```python
from build123d import *

# Parameters (mm, degrees)
F0_W      = 79.3684571981
F0_H      = 71.8531981111
F1_DEPTH  = 25.4
F2_DEPTH  = 25.4
F4_DEPTH  = 101.6
F5_R      = 4.7587178315
F6_DEPTH  = 127
F7_DEPTH  = 508
F9_DEPTH  = 7.62
F11_DEPTH = 25.4
F12_DEPTH = 12.7


with BuildPart() as f1:
    # F0 (on Top) → F1 (new body)
    with BuildSketch(Plane.XY):
        Rectangle(F0_W, F0_H)
    extrude(amount=F1_DEPTH)

    # F2 (add): a face of the model
    f2_faces = [f1.faces().sort_by_distance(p)[0] for p in [
        (0, 0, 25.4),
    ]]
    extrude(f2_faces, amount=F2_DEPTH)

    # F3 (on face) → F4 (cut)
    with BuildSketch(Plane.XZ.offset(35.9265990555)):
        with BuildLine():
            ThreePointArc((-17.4702548625, 50.8), (0, 33.3297451375), (17.4702548625, 50.8))
            Line((17.4702548625, 50.8), (-17.4702548625, 50.8))
        make_face()
    extrude(amount=-F4_DEPTH, mode=Mode.SUBTRACT)

    # F5 (on face) → F6 (join)
    with BuildSketch(Plane.XY.offset(50.8)):
        with Locations((-29.7860819846, 0)):
            Circle(F5_R)
        with Locations((28.1363911927, 0)):
            Circle(F5_R)
    extrude(amount=F6_DEPTH)

    # F7 (cut): faces of the model
    f7_faces = [f1.faces().sort_by_distance(p)[0] for p in [
        (28.1363911927, 0, 177.8),
        (-29.7860819846, 0, 177.8),
    ]]
    extrude(f7_faces, amount=-F7_DEPTH, mode=Mode.SUBTRACT)

    # F8 (on face) → F9 (join)
    with BuildSketch(Plane.XZ.offset(35.9265990555)):
        with BuildLine():
            Line((-17.4702548625, 50.8), (-22.6149617575, 50.8))
            ThreePointArc((-22.6149617575, 50.8), (0, 28.1850382425), (22.6149617575, 50.8))
            Line((22.6149617575, 50.8), (17.4702548625, 50.8))
            ThreePointArc((17.4702548625, 50.8), (0, 33.3297451375), (-17.4702548625, 50.8))
        make_face()
    extrude(amount=F9_DEPTH)

    # F10 (on face) → F11 (join)
    with BuildSketch(Plane(origin=(0, 35.9265990555, 0), x_dir=(-1, 0, 0), z_dir=(0, 1, 0))):
        with BuildLine():
            Line((-17.4702548625, 50.8), (-23.0630593563, 50.8))
            ThreePointArc((-23.0630593563, 50.8), (0, 27.7369406437), (23.0630593563, 50.8))
            Line((23.0630593563, 50.8), (17.4702548625, 50.8))
            ThreePointArc((17.4702548625, 50.8), (0, 33.3297451375), (-17.4702548625, 50.8))
        make_face()
    extrude(amount=F11_DEPTH)

    # F12 (cut): a face of the model
    f12_faces = [f1.faces().sort_by_distance(p)[0] for p in [
        (20.2666571094, 61.3265990555, 50.2842943151),
    ]]
    extrude(f12_faces, amount=-F12_DEPTH, mode=Mode.SUBTRACT)


solid = f1.part
```
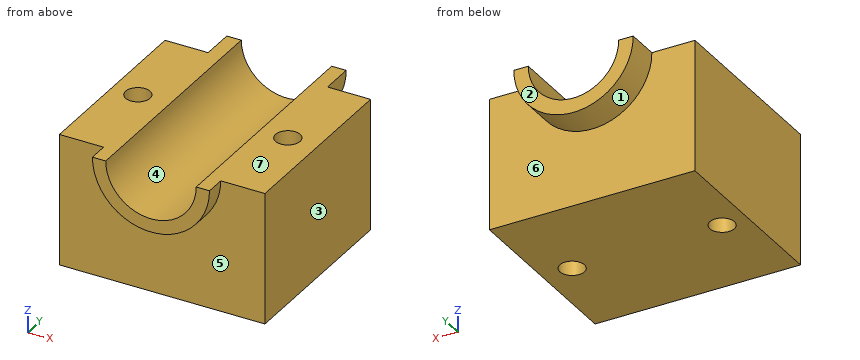
Check sheet for the modelled part. Datum: model origin and axes. Units: mm. Face numbers are marked on the shaded views. A direction names the side the tool comes from. Coordinates: 2 decimals unless noted, no trailing zeros. Order: outer loops, then holes, each group sorted by start corner. A loop starts at its lowest first (then second) coordinate and runs counter-clockwise, first axis right, second up. Notation, with made-up numbers: M 20,82 L 56,82 A10 ccw 56,97 Z; hole C -14,9.25 d5. An arc over 180 degrees is marked long. One line per question, with ' | ' between items. Start each with the question number.
Item 1: Access from +Z, -Z, +X, -X, +Y, -Y to the whole of each face (thin tool, end or side, straight path). Record for the marked faces 5, 6 and 7.
Item 2: Sectioned sample at A-A on y = 0. Record the cut outline in (x, z).
Item 3: Gauge pin test, flat ends, axial feed: P1, Ø15, axis at x = 14.5, z = 13, coming from the +Y side; P2, Ø1.5, axis at x = -30, z = 35, coming from the -Y side. Record the tip position at first contact, or that the pin passes through.
Item 4: Sectioned sample at D-D on x = -6. Record the cut outline in (y, z), and give its area (3 significant figures).
Item 5: Material ranges on line 1 (Y direction, x = -6, z = 19); line 2 (X direction, y = 45, z = 41.5); line 3 (X direction, y = -29.5, z = 38), recorded low to high.
Item 6: Sectioned sample at B-B on z = 38. Record the cut outline in (x, y), and give its area (3 significant figures).
Item 7: Sectioned sample at C-C on y = -34.5. Record the cut outline in (x, z), and give its area (3 significant figures).
Item 8: Mould release check, pull along X, two halves, no side actions. Record for the marked faces 1, 2, 3 and 4: pulls with the +X half, pulls with the -X half, needs draft (parallel to the pull), parting line crosses it, or undercut.
Answer below:
1) face 5: -Z, -Y | face 6: -Z, +Y | face 7: +Z, +X, -X, +Y, -Y
2) outline: M -39.68,0 L -34.54,0 L -34.54,50.8 L -39.68,50.8 Z; M -25.03,0 L 23.38,0 L 23.38,50.8 L 17.47,50.8 A17.47 cw -17.47,50.8 L -25.03,50.8 Z; M 32.9,0 L 39.68,0 L 39.68,50.8 L 32.9,50.8 Z
3) P1: stops at y = 35.93 | P2: stops at y = -35.93
4) outline: M -43.55,29 L -35.93,29 L -35.93,0 L 35.93,0 L 35.93,28.53 L 48.63,28.53 L 48.63,34.39 L -43.55,34.39 Z | area: 2,590 mm^2
5) line 1: y = -35.93 to 35.93 | line 2: x = -21.1 to -14.79, 14.79 to 21.1 | line 3: x = -39.68 to -11.89, 11.89 to 39.68
6) outline: M -39.68,-35.93 L -18.64,-35.93 L -18.64,-43.55 L -11.89,-43.55 L -11.89,48.63 L -19.19,48.63 L -19.19,35.93 L -39.68,35.93 Z; M 11.89,-43.55 L 18.64,-43.55 L 18.64,-35.93 L 39.68,-35.93 L 39.68,35.93 L 19.19,35.93 L 19.19,48.63 L 11.89,48.63 Z; hole C -29.79,0 d9.52; hole C 28.14,0 d9.52 | area: 4,140 mm^2
7) outline: M -39.68,0 L 39.68,0 L 39.68,50.8 L 17.47,50.8 A17.47 cw -17.47,50.8 L -39.68,50.8 Z | area: 3,550 mm^2
8) face 1: parting line crosses it | face 2: needs draft | face 3: pulls with the +X half | face 4: undercut
